Here's how the part is built. I have some questions about the finished solid (model axes, mm). A direction names the side the tool comes from. Round coordinates to 2 decimals unless told otherwise and drop trailing zeros. Order: outer loops, then holes, each group sorted by start corner. A loop starts at its lowest first (then second) coordinate and runs counter-clockwise, first axis right, second up. Notation, with made-up numbers: (10, 80) -> (57, 80) arc R20 cw to (57, 89) -> close; hole circle Ø1 at (-37.5, 38). An arc over 180 degrees is marked (long way). Answer in a Markdown table with one row per item.
```python
from build123d import *

# Parameters (mm, degrees)
F0_W     = 441
F0_H     = 210
F1_DEPTH = 44
F2_T     = -0.5
F4_DEPTH = 44
F7_DEPTH = 3


with BuildPart() as f1:
    # F0 (on Top) → F1 (new body)
    with BuildSketch(Plane.XY):
        Rectangle(F0_W, F0_H)
    extrude(amount=F1_DEPTH)

    # F2
    f2_openings = [f1.faces().sort_by_distance(p)[0] for p in [
        (0, 0, 44),
    ]]
    offset(amount=F2_T, openings=f2_openings)


with BuildPart() as f4:
    # F3 (on face) → F4 (new body)
    with BuildSketch(Plane(origin=(0, 0, 0), x_dir=(1, 0, 0), z_dir=(0, 0, -1))):
        Polygon((-223.5, 55), (-220.5, 55), (-220.5, 105), (-240.5, 105), (-240.5, 102), (-223.5, 102), align=None)
        Polygon((220.5, 55), (223.5, 55), (223.5, 102), (240.5, 102), (240.5, 105), (220.5, 105), align=None)
    extrude(amount=-F4_DEPTH)

    # F5: union F1
    add(f1.part)

    # F6 (on face) → F7 (cut)
    with BuildSketch(Plane.XZ.offset(105)):
        with BuildLine():
            Line((-234.112281, 37.43943), (-233.890185, 37.439508))
            ThreePointArc((-233.890185, 37.439508), (-234.001233, 37.441231), (-234.112281, 37.43943))
        make_face()
        with BuildLine():
            Line((-229.001233, 37.441231), (-233.890185, 37.439508))
            Line((-233.890185, 37.439508), (-234.112281, 37.43943))
            ThreePointArc((-234.112281, 37.43943), (-237.499245, 33.868521), (-233.966869, 30.441388))
            Line((-233.966869, 30.441388), (-229.000111, 30.441232))
            ThreePointArc((-229.000111, 30.441232), (-225.5, 33.941793), (-229.001233, 37.441231))
        make_face()
        with BuildLine():
            Line((-229.000111, 13.558768), (-233.966869, 13.558612))
            ThreePointArc((-233.966869, 13.558612), (-237.499245, 10.131479), (-234.112281, 6.56057))
            Line((-234.112281, 6.56057), (-233.890185, 6.560492))
            Line((-233.890185, 6.560492), (-229.001233, 6.558769))
            ThreePointArc((-229.001233, 6.558769), (-225.5, 10.058207), (-229.000111, 13.558768))
        make_face()
        with BuildLine():
            Line((-233.890185, 6.560492), (-234.112281, 6.56057))
            ThreePointArc((-234.112281, 6.56057), (-234.001233, 6.558769), (-233.890185, 6.560492))
        make_face()
        with BuildLine():
            ThreePointArc((233.966869, 30.441388), (237.499245, 33.868521), (234.112281, 37.43943))
            Line((234.112281, 37.43943), (233.890185, 37.439508))
            Line((233.890185, 37.439508), (229.001233, 37.441231))
            ThreePointArc((229.001233, 37.441231), (225.5, 33.941793), (229.000111, 30.441232))
            Line((229.000111, 30.441232), (233.966869, 30.441388))
        make_face()
        with BuildLine():
            Line((233.890185, 37.439508), (234.112281, 37.43943))
            ThreePointArc((234.112281, 37.43943), (234.001233, 37.441231), (233.890185, 37.439508))
        make_face()
        with BuildLine():
            ThreePointArc((234.112281, 6.56057), (237.499245, 10.131479), (233.966869, 13.558612))
            Line((233.966869, 13.558612), (229.000111, 13.558768))
            ThreePointArc((229.000111, 13.558768), (225.5, 10.058207), (229.001233, 6.558769))
            Line((229.001233, 6.558769), (233.890185, 6.560492))
            Line((233.890185, 6.560492), (234.112281, 6.56057))
        make_face()
        with BuildLine():
            ThreePointArc((233.890185, 6.560492), (234.001233, 6.558769), (234.112281, 6.56057))
            Line((234.112281, 6.56057), (233.890185, 6.560492))
        make_face()
    extrude(amount=-F7_DEPTH, mode=Mode.SUBTRACT)


solid = f4.part
```
1. For pin 1 Ø3 at (y, z) = (-80, 10) entering from +X; pin 2 Ø10 at (x, y) = (49.5, -49.5) entering from +Z; pin 3 Ø5 at (x, z) = (-228.5, 18) entering from +Y, each with a flat end and sliding along its axis, tell me the tip position at first contact or that it passes through.
Numbers:
| item | result |
|---|---|
| pin 1 | stops at x = 223.5 |
| pin 2 | stops at z = 0.5 |
| pin 3 | stops at y = -102 |
2. Please list where these lines run through material, in increasing order: line 1 along X through (y, z) = (43, 25); line 2 along Y through (x, z) = (59.5, 20.5); line 3 along X through (y, z) = (-71, 40).
Numbers:
| item | result |
|---|---|
| line 1 | x = -220.5 to -220, 220 to 220.5 |
| line 2 | y = -105 to -104.5, 104.5 to 105 |
| line 3 | x = -223.5 to -220, 220 to 223.5 |
3. We'd pull the mould along Y, two halves only. Please class faces 1 (the face through (-3, 105, 22)), 2 (the face through (220.5, 24, 22)), 3 (the face through (-220, -1, 22)), 4 (the face through (-3, 1, 0.5)): released by +Y, released by -Y, zero draft, split by the parting line, or undercut.
Numbers:
| item | result |
|---|---|
| face 1 | released by +Y |
| face 2 | zero draft |
| face 3 | undercut |
| face 4 | undercut |
4. For faces 5 (the face through (-3, -104.5, 22)), 6 (the face through (232, -102, 22)), 7 (the face through (-223.5, -79, 22)), which set-ups out of +Z, -Z, +X, -X, +Y, -Y let a thin tool reach every point of the face, with its end or its side?
Numbers:
| item | result |
|---|---|
| face 5 | +Z |
| face 6 | +Z, -Z, +X, +Y |
| face 7 | +Z, -Z, -X, +Y |
5. Suppose I cut it at C-C on y = -84. Write out the boundary of the cut face in (x, z), then the cut area to 3 significant figures.
Numbers:
| item | result |
|---|---|
| outline | (-223.5, 0) -> (223.5, 0) -> (223.5, 44) -> (220, 44) -> (220, 0.5) -> (-220, 0.5) -> (-220, 44) -> (-223.5, 44) -> close |
| area | 528 mm2 |
6. Suppose I cut it at A-A on z = 25. Write out the boundary of the cut face in (x, y).
Numbers:
| item | result |
|---|---|
| outline | (-240.5, -105) -> (240.5, -105) -> (240.5, -102) -> (223.5, -102) -> (223.5, -55) -> (220.5, -55) -> (220.5, 105) -> (-220.5, 105) -> (-220.5, -55) -> (-223.5, -55) -> (-223.5, -102) -> (-240.5, -102) -> close; hole (-220, -104.5) -> (220, -104.5) -> (220, 104.5) -> (-220, 104.5) -> close |
7. Suppose I cut it at B-B on x = 201.5. Write out the boundary of the cut face in (y, z), then the cut area to 4 significant figures.
Numbers:
| item | result |
|---|---|
| outline | (-105, 0) -> (105, 0) -> (105, 44) -> (104.5, 44) -> (104.5, 0.5) -> (-104.5, 0.5) -> (-104.5, 44) -> (-105, 44) -> close |
| area | 148.5 mm2 |
